```python
from build123d import *

# Parameters (mm, degrees)
PROFILE_DEPTH         = 1
USBCCUTOUT_DEPTH      = 7.385922016
USBCCUTOUT_DEPTH_BACK = 7.385922016


with BuildPart() as part:
    # ProfileS → Profile (new, symmetric)
    with BuildSketch(Plane.XY):
        with BuildLine():
            Line((-3, 2.7), (3, 2.7))
            ThreePointArc((3, 2.7), (5.7, 0), (3, -2.7))
            Line((3, -2.7), (-3, -2.7))
            ThreePointArc((-3, -2.7), (-5.7, 0), (-3, 2.7))
        make_face()
    extrude(amount=PROFILE_DEPTH, both=True)

    # USBCCutoutS → USBCCutout (cut, two sides: drawn at the far end of the back side and taken through both)
    with BuildSketch(Plane.XY.offset(-USBCCUTOUT_DEPTH_BACK)):
        with BuildLine():
            Line((-2.95, 1.2), (2.95, 1.2))
            ThreePointArc((2.95, 1.2), (4.15, 0), (2.95, -1.2))
            Line((2.95, -1.2), (-2.95, -1.2))
            ThreePointArc((-2.95, -1.2), (-4.15, 0), (-2.95, 1.2))
        make_face()
    extrude(amount=USBCCUTOUT_DEPTH + USBCCUTOUT_DEPTH_BACK, mode=Mode.SUBTRACT)


solid = part.part
```
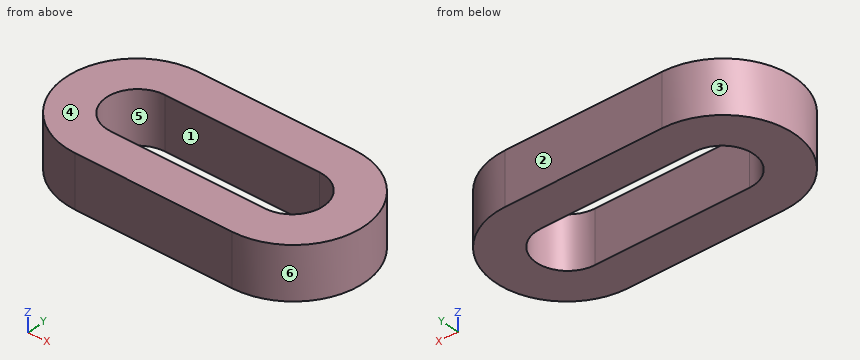
Design review of the part built by this model. Coordinates are the model's own, in mm. Face numbers are marked on the shaded views. A direction names the side the tool comes from. Round coordinates to 2 decimals unless told otherwise and drop trailing zeros. Write each loop counter-clockwise with the first axis right and the second up, starting at its lowest first coordinate (ties: lowest second). Pieces come first, ordered by that corner, then holes.
Item 1: We need section B-B on y = 0. Write out the cut boundary in (x, z), and give its area (3 significant figures).
Item 2: We need section A-A on x = 2.5. Write out the cut boundary in (y, z).
Item 3: The part is to be moulded in two halves that separate along X. For the marked faces 3, 4, 5 and 6, say which applies: +X half, -X half, draft (parallel to the pull), parting line (faces both ways), or undercut.
Item 4: For the marked faces 1 and 2, list the 3-axis set-ups (+Z, -Z, +X, -X, +Y, -Y) from which the entire face can be reached by the end or side of a thin tool; tool diameter is ignored.
Item 5: For probe 1 along Y at (x, z) = (0, -0.3); probe 2 along Y at (x, z) = (-4, 0.85); probe 3 along X at (y, z) = (-0.15, 0.8), list the stretches that pass through material, from the lowest coordinate up.
Item 6: We need section C-C on z = 0.45. Write out the cut boundary in (x, y).
Item 7: We need section D-D on x = 4.5. Write out the cut boundary in (y, z) (3 decimals).
Returned:
1. outline: (-5.7, -1) - (-4.15, -1) - (-4.15, 1) - (-5.7, 1) - close; (4.15, -1) - (5.7, -1) - (5.7, 1) - (4.15, 1) - close
1. area: 6.20 mm2
2. outline: (-2.7, -1) - (-1.2, -1) - (-1.2, 1) - (-2.7, 1) - close; (1.2, -1) - (2.7, -1) - (2.7, 1) - (1.2, 1) - close
3. face 3: -X half
3. face 4: draft
3. face 5: undercut
3. face 6: +X half
4. face 1: +Z, -Z
4. face 2: +Z, -Z, +X, -X, +Y
5. probe 1: y = -2.7 to -1.2, 1.2 to 2.7
5. probe 2: y = -2.51 to -0.58, 0.58 to 2.51
5. probe 3: x = -5.7 to -4.14, 4.14 to 5.7
6. outline: (-3, -2.7) - (3, -2.7) arc R2.7 ccw to (3, 2.7) - (-3, 2.7) arc R2.7 ccw to start; hole (-2.95, -1.2) - (2.95, -1.2) arc R1.2 ccw to (2.95, 1.2) - (-2.95, 1.2) arc R1.2 ccw to start
7. outline: (-2.245, -1) - (2.245, -1) - (2.245, 1) - (-2.245, 1) - close
